Verification items for the finished model (mm, model axes). A direction names the side the tool comes from. Coordinates: 2 decimals unless noted, no trailing zeros. Order: outer loops, then holes, each group sorted by start corner. A loop starts at its lowest first (then second) coordinate and runs counter-clockwise, first axis right, second up.
Q1. Set-up check for faces 4 (the cylindrical face through (2.51, 5.79, -203.33)), 5 (the cylindrical face through (84.77, 44.903, 210.58)), 6 (the flat face through (3, 89, 209.55)), 7 (the cylindrical face through (0.838, -1.03, -48.777)), 8 (the cylindrical face through (-171.749, 107.057, 210.58)): record each of +Z, -Z, +X, -X, +Y, -Y from which the full face is reachable in a straight line by a thin tool's end or side.
Q2. Cross-section at A-A, the plane z = 11.5. Record the boundary of the cut face in (x, y), and give its area (3 significant figures).
Q3. Cross-section at C-C, the plane x = 0. Record the boundary of the cut face in (y, z).
Q4. Cross-section at B-B, the plane x = 88.9. Record the boundary of the cut face in (y, z), and give its area (3 significant figures).
Q5. Cross-section at D-D, the plane y = 63.5. Record the boundary of the cut face in (x, z), and give its area (3 significant figures).
Q6. Thickness scan on line 1 (X direction, y = 63, z = 210); line 2 (Z direction, x = 107, y = 23.5); line 3 (Z direction, x = 138, y = 48). Record the ranges inside material, lowest first.
Q7. Depth check by flat-ended pin: P1, Ø12, axis at x = 93, y = 54, coming from the +Z side; P2, Ø1.6, axis at x = -20, z = 210.5, coming from the +Y side; P3, Ø2, axis at x = -27.5, y = -1, coming from the -Z side. Enter the tip coordinate at first touch or a pass-through.
Q8. Draft check along X on faces 1 (the cylindrical face through (-124.77, -1.03, 157.16)), 2 (the cylindrical face through (171.749, 107.057, 210.58)), 3 (the flat face through (3, 90, 211.582)). Enter one of: pulls with the +X half, pulls with the -X half, needs draft (parallel to the pull), parting line crosses it, or undercut.
from build123d import *

# Parameters (mm, degrees)
F1_DEPTH  = 179.3875
F2_R      = 25.4
F4_DEPTH  = 2.032
F6_DEPTH  = 2.032
F8_DEPTH  = 2.54
F9_R      = 25.4
F10_DEPTH = 25.4
F11_R     = 19.05
F12_DEPTH = 25.4


with BuildPart() as f1:
    # F0 (on Right) → F1 (new body, symmetric)
    with BuildSketch(Plane.YZ):
        with BuildLine():
            Line((0, -184.15), (0, 184.15))
            ThreePointArc((0, 184.15), (7.439488, 202.110512), (25.4, 209.55))
            Line((25.4, 209.55), (114.3, 209.55))
            Line((114.3, 209.55), (114.3, 211.582))
            Line((114.3, 211.582), (25.4, 211.582))
            ThreePointArc((25.4, 211.582), (6.002647, 203.547353), (-2.032, 184.15))
            Line((-2.032, 184.15), (-2.032, -184.15))
            ThreePointArc((-2.032, -184.15), (6.002647, -203.547353), (25.4, -211.582))
            Line((25.4, -211.582), (182.88, -211.582))
            Line((182.88, -211.582), (182.88, -209.55))
            Line((182.88, -209.55), (25.4, -209.55))
            ThreePointArc((25.4, -209.55), (7.439488, -202.110512), (0, -184.15))
        make_face()
    extrude(amount=F1_DEPTH, both=True)

    # F2
    f2_edges = [f1.edges().sort_by_distance(p)[0] for p in [
        (179.3875, 114.3, 210.566),
        (-179.3875, 114.3, 210.566),
        (-179.3875, 182.88, -210.566),
        (179.3875, 182.88, -210.566),
    ]]
    fillet(f2_edges, radius=F2_R)

    # F3 (on face) → F4 (cut)
    with BuildSketch(Plane.XZ.offset(2.032)):
        with BuildLine():
            Line((115.8875, 160.782), (-115.8875, 160.782))
            ThreePointArc((-115.8875, 160.782), (-124.867756, 157.062256), (-128.5875, 148.082))
            Line((-128.5875, 148.082), (-128.5875, -17.018))
            ThreePointArc((-128.5875, -17.018), (-124.867756, -25.998256), (-115.8875, -29.718))
            Line((-115.8875, -29.718), (115.8875, -29.718))
            ThreePointArc((115.8875, -29.718), (124.867756, -25.998256), (128.5875, -17.018))
            Line((128.5875, -17.018), (128.5875, 148.082))
            ThreePointArc((128.5875, 148.082), (124.867756, 157.062256), (115.8875, 160.782))
        make_face()
    extrude(amount=-F4_DEPTH, mode=Mode.SUBTRACT)

    # F5 (on face) → F6 (cut)
    with BuildSketch(Plane.XZ.offset(2.032)):
        with BuildLine():
            Line((38.1, -99.568), (38.1, -86.868))
            ThreePointArc((38.1, -86.868), (0, -48.768), (-38.1, -86.868))
            Line((-38.1, -86.868), (-38.1, -99.568))
            ThreePointArc((-38.1, -99.568), (0, -137.668), (38.1, -99.568))
        make_face()
    extrude(amount=-F6_DEPTH, mode=Mode.SUBTRACT)

    # F7 (on face) → F8 (cut)
    with BuildSketch(Plane.XZ.offset(2.032)):
        with BuildLine():
            ThreePointArc((142.875, 1.7145), (141.2875, 3.302), (139.7, 1.7145))
            Line((139.7, 1.7145), (139.7, -20.5105))
            ThreePointArc((139.7, -20.5105), (141.2875, -22.098), (142.875, -20.5105))
            Line((142.875, -20.5105), (142.875, 1.7145))
        make_face()
        with BuildLine():
            ThreePointArc((-139.7, 1.7145), (-141.2875, 3.302), (-142.875, 1.7145))
            Line((-142.875, 1.7145), (-142.875, -20.5105))
            ThreePointArc((-142.875, -20.5105), (-141.2875, -22.098), (-139.7, -20.5105))
            Line((-139.7, -20.5105), (-139.7, 1.7145))
        make_face()
    extrude(amount=-F8_DEPTH, mode=Mode.SUBTRACT)

    # F9 (on face) → F10 (cut)
    with BuildSketch(Plane.XY.offset(211.582)):
        with Locations((0, 63.5)):
            Circle(F9_R)
    extrude(amount=-F10_DEPTH, mode=Mode.SUBTRACT)

    # F11 (on face) → F12 (cut)
    with BuildSketch(Plane.XY.offset(211.582)):
        with Locations((88.9, 63.5)):
            Circle(F11_R)
    extrude(amount=-F12_DEPTH, mode=Mode.SUBTRACT)


solid = f1.part
Check values:
1. face 4: -Z, +X, -X, -Y
1. face 5: +Z
1. face 6: +X, -X, +Y
1. face 7: +Y, -Y
1. face 8: +Z, -X, +Y
2. outline: (-179.39, -2.03) - (-128.59, -2.03) - (-128.59, 0) - (-179.39, 0) - close; (128.59, -2.03) - (179.39, -2.03) - (179.39, 0) - (128.59, 0) - close
2. area: 206 mm2
3. outline: (-2.03, -184.15) arc R27.43 ccw to (25.4, -211.58) - (182.88, -211.58) - (182.88, -209.55) - (25.4, -209.55) arc R25.4 cw to (0, -184.15) - (0, -137.67) - (-2.03, -137.67) - close; (-2.03, -48.77) - (0, -48.77) - (0, -29.72) - (-2.03, -29.72) - close; (-2.03, 160.78) - (0, 160.78) - (0, 184.15) arc R25.4 cw to (25.4, 209.55) - (38.1, 209.55) - (38.1, 211.58) - (25.4, 211.58) arc R27.43 ccw to (-2.03, 184.15) - close; (88.9, 209.55) - (114.3, 209.55) - (114.3, 211.58) - (88.9, 211.58) - close
4. outline: (-2.03, -184.15) arc R27.43 ccw to (25.4, -211.58) - (182.88, -211.58) - (182.88, -209.55) - (25.4, -209.55) arc R25.4 cw to (0, -184.15) - (0, -29.72) - (-2.03, -29.72) - close; (-2.03, 160.78) - (0, 160.78) - (0, 184.15) arc R25.4 cw to (25.4, 209.55) - (44.45, 209.55) - (44.45, 211.58) - (25.4, 211.58) arc R27.43 ccw to (-2.03, 184.15) - close; (82.55, 209.55) - (114.3, 209.55) - (114.3, 211.58) - (82.55, 211.58) - close
4. area: 953 mm2
5. outline: (-179.39, -211.58) - (179.39, -211.58) - (179.39, -209.55) - (-179.39, -209.55) - close; (-179.39, 209.55) - (-25.4, 209.55) - (-25.4, 211.58) - (-179.39, 211.58) - close; (25.4, 209.55) - (69.85, 209.55) - (69.85, 211.58) - (25.4, 211.58) - close; (107.95, 209.55) - (179.39, 209.55) - (179.39, 211.58) - (107.95, 211.58) - close
5. area: 1,280 mm2
6. line 1: x = -179.39 to -25.4, 25.4 to 69.86, 107.94 to 179.39
6. line 2: z = -211.52 to -209.48, 209.48 to 211.52
6. line 3: z = -211.58 to -209.55, 209.55 to 211.58
7. P1: stops at z = -209.55
7. P2: stops at y = 114.3
7. P3: stops at z = -194.51
8. face 1: undercut
8. face 2: pulls with the +X half
8. face 3: needs draft
